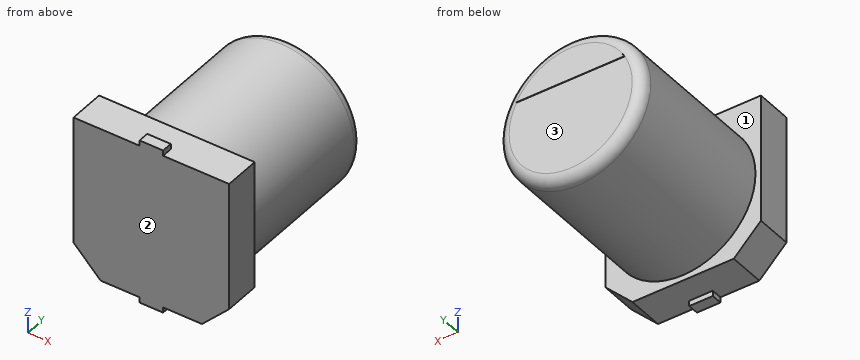
from build123d import *

# Parameters (mm, degrees)
BOSS_EXTRUDE1_DEPTH = 1
SKETCH3_R           = 2
BOSS_EXTRUDE2_DEPTH = 5.4
FILLET1_R           = 0.3
SKETCH4_W           = 0.65
SKETCH4_H           = 1.8
BOSS_EXTRUDE3_DEPTH = 0.3
BOSS_EXTRUDE4_DEPTH = 0.01


with BuildPart() as part:
    # Sketch2 → Boss-Extrude1 (new body)
    with BuildSketch(Plane(origin=(0, 0, 0), x_dir=(1, 0, 0), z_dir=(0, 1, 0))):
        Polygon((2.15, -2.15), (-2.15, -2.15), (-2.15, 1.4), (-1.4, 2.15), (1.4, 2.15), (2.15, 1.4), align=None)
    extrude(amount=BOSS_EXTRUDE1_DEPTH)

    # Sketch3 → Boss-Extrude2 (add)
    with BuildSketch(Plane(origin=(0, 0, 0), x_dir=(1, 0, 0), z_dir=(0, 1, 0))):
        Circle(SKETCH3_R)
    extrude(amount=BOSS_EXTRUDE2_DEPTH)

    # Fillet1
    fillet1_edges = [part.edges().sort_by_distance(p)[0] for p in [
        (-2, 5.4, 0),
    ]]
    fillet(fillet1_edges, radius=FILLET1_R)

    # Sketch4 → Boss-Extrude3 (add)
    with BuildSketch(Plane(origin=(0, 0, 0), x_dir=(1, 0, 0), z_dir=(0, 1, 0))):
        with Locations((0, 1.4)):
            Rectangle(SKETCH4_W, SKETCH4_H)
        with Locations((0, -1.4)):
            Rectangle(SKETCH4_W, SKETCH4_H)
    extrude(amount=BOSS_EXTRUDE3_DEPTH)

    # Sketch5 → Boss-Extrude4 (add)
    with BuildSketch(Plane(origin=(0, 5.4, 0), x_dir=(1, 0, 0), z_dir=(0, 1, 0))):
        with BuildLine():
            Line((1.493037561, -0.812919948), (-1.493037561, -0.812919948))
            ThreePointArc((-1.493037561, -0.812919948), (0, -1.7), (1.493037561, -0.812919948))
        make_face()
    extrude(amount=BOSS_EXTRUDE4_DEPTH)


solid = part.part
The model under review builds one solid part; all positions refer to its coordinate system, in mm. Face numbers are marked on the shaded views. A direction names the side the tool comes from. Give positions to 0.01 mm unless a question says otherwise; leave off trailing zeros. Order: outer loops, then holes, each group sorted by start corner. A loop starts at its lowest first (then second) coordinate and runs counter-clockwise, first axis right, second up. Notation, with made-up numbers: M -29.75,82.25 L 4.25,82.25 A31 cw 4.25,114.25 Z; hole C 37.5,-27 d8. An arc over 180 degrees is marked long. Answer in a Markdown table with one row per item. Add a question column.
1. For pin 1 Ø2 at (y, z) = (1.5, -1.5) entering from +X; pin 2 Ø1.5 at (x, z) = (0.5, 0) entering from +Y; pin 3 Ø1 at (x, y) = (-0.5, 2.5) entering from -Z, all flat-tipped, find the tip position at first contact; note any pin that passes through.
2. Add section C-C on y = 3.7. State the section outline as (x, z) points, plus the area to 3 significant figures.
3. To check wall thickness, follow line 1 along Y through (x, z) = (1.4, -0.05); line 2 along Y through (x, z) = (-1.65, 1.2); line 3 along Z through (x, y) = (0.35, 2.95). State the ranges of each line that lie inside material, in increasing order.
4. Add section A-A on z = 0. State the section outline as (x, y) points.
5. Machinability: for the marked faces 1, 2 and 3, which of the approach directions +Z, -Z, +X, -X, +Y, -Y give a long, thin tool a straight path to every point of the face, cutting with its end or side? Answer none if there is none.
The answers:
| question | item | result |
|---|---|---|
| 1 | pin 1 | x = 2.15 |
| 1 | pin 2 | y = 5.4 |
| 1 | pin 3 | z = -2 |
| 2 | outline | C 0,0 d4 |
| 2 | area | 12.6 mm2 |
| 3 | line 1 | 0 to 5.4 |
| 3 | line 2 | 0 to 1 |
| 3 | line 3 | -1.97 to 1.97 |
| 4 | outline | M -2.15,0 L 2.15,0 L 2.15,1 L 2,1 L 2,5.1 A0.3 ccw 1.7,5.4 L -1.7,5.4 A0.3 ccw -2,5.1 L -2,1 L -2.15,1 Z |
| 5 | face 1 | +Y |
| 5 | face 2 | +Z, -Z, +X, -X, -Y |
| 5 | face 3 | -Z, +X, -X, +Y |
